Can you work these out from the model? Positions are in its coordinate system, mm. A direction names the side the tool comes from. Coordinates: 2 decimals unless noted, no trailing zeros. Loops run counter-clockwise (first coordinate to the right, second up) from the corner with the lowest first, then second, coordinate; pieces in that order, holes last. Notation, with made-up numbers: M -13.75,-0.5 L 29.25,-0.5 A25 ccw 29.25,25.5 Z; hole C -14,6.25 d6. An arc over 180 degrees is marked long. Answer as a JSON object with one key per item and string values. Group by question number.
Item 1: I'm going to push flat-ended pins straight in: pin 1 Ø5 at (x, y) = (3.5, 69.5) entering from +Z; pin 2 Ø10 at (y, z) = (7, 0) entering from -X; pin 3 Ø5 at (y, z) = (16, 0) entering from +X; pin 4 Ø12 at (x, y) = (-5, 34) entering from -Z. Where does each tip first touch, or does it pass through?
Item 2: Suppose I cut it at C-C (y = 69). Write out the boundary of the cut face in (x, z).
Item 3: Suppose I cut it at B-B (y = 19.5). Write out the boundary of the cut face in (x, z), then the cut area to 3 significant figures.
Item 4: If I drill on line 1 (Y direction, x = 18, z = -5.5); line 2 (Z direction, x = 10, y = 5); line 3 (Y direction, x = -1, z = 9), over which ranges is the centre line in solid material (lowest first)?
Item 5: Which directions (+Z, -Z, +X, -X, +Y, -Y) give clear straight access to the entire face, cutting with the end or side of a thin tool? Please do faces 4 (the cylindrical face through (-0.9, -0.99, -2.86)), 5 (the cylindrical face through (-7.509, 22.717, -23.846)), 6 (the flat face through (15, 45, 0)).
Item 6: We'd pull the mould along X, two halves only. Please class faces 1 (the cylindrical face through (-0.228, 4.93, 11.735)), 2 (the cylindrical face through (12.4, 48.5, -6.5)), 3 (the flat face through (0, -2, 0)): +X half, -X half, draft (parallel to the pull), parting line (faces both ways), or undercut.
Item 7: Suppose I cut it at A-A (x = 0). Write out the boundary of the cut face in (y, z).
```python
from build123d import *

# Parameters (mm, degrees)
SKETCH1_W          = 3
SKETCH1_H          = 2
SKETCH1_W_2        = 4
SKETCH1_H_2        = 7
SKETCH1_W_3        = 10
SKETCH1_H_3        = 28
CHAMFER1_SIZE      = 7
CHAMFER1_SIZE2     = 2.54779164
CHAMFER2_SIZE      = 7
CHAMFER2_SIZE2     = 2.54779164
SKETCH2_R          = 1.75
CUT_EXTRUDE1_DEPTH = 10


with BuildPart() as part:
    # Sketch1 → Revolve1 (revolve)
    with BuildSketch(Plane.XY, mode=Mode.PRIVATE) as revolve1_sk:
        Polygon((0, 45), (0, 0), (3, 0), (25, 0), (25, 45), (14, 45), (4, 45), align=None)
        with Locations((1.5, -1)):
            Rectangle(SKETCH1_W, SKETCH1_H)
        with Locations((2, 48.5)):
            Rectangle(SKETCH1_W_2, SKETCH1_H_2)
        with Locations((9, 48.5)):
            Rectangle(SKETCH1_W_3, SKETCH1_H_2)
        with Locations((2, 66)):
            Rectangle(SKETCH1_W_2, SKETCH1_H_3)
    revolve(revolve1_sk.sketch.rotate(Axis((0, 45, 0), (0, 1, 0)), 90), axis=Axis((0, 45, 0), (0, 1, 0)))

    # Chamfer1
    chamfer1_edges = [part.edges().sort_by_distance(p)[0] for p in [
        (0, 0, 25),
    ]]
    chamfer1_side = [part.faces().sort_by_distance(p)[0] for p in [
        (0, 22.5, 25),
    ]]
    chamfer(chamfer1_edges, length=CHAMFER1_SIZE, length2=CHAMFER1_SIZE2, reference=chamfer1_side[0])

    # Chamfer2
    chamfer2_edges = [part.edges().sort_by_distance(p)[0] for p in [
        (0, 45, 25),
    ]]
    chamfer2_side = [part.faces().sort_by_distance(p)[0] for p in [
        (0, 26, 25),
    ]]
    chamfer(chamfer2_edges, length=CHAMFER2_SIZE, length2=CHAMFER2_SIZE2, reference=chamfer2_side[0])

    # Sketch2 → Cut-Extrude1 (cut)
    with BuildSketch(Plane.XZ):
        with Locations((0, 10)):
            Circle(SKETCH2_R)
        with Locations((10, 0)):
            Circle(SKETCH2_R)
        with Locations((0, -10)):
            Circle(SKETCH2_R)
        with Locations((-10, 0)):
            Circle(SKETCH2_R)
    extrude(amount=-CUT_EXTRUDE1_DEPTH, mode=Mode.SUBTRACT)


solid = part.part
```
From the geometry:
{
 "1": {"pin 1": "z = 3.87", "pin 2": "x = -25", "pin 3": "x = 25", "pin 4": "z = -25"},
 "2": {"outline": "C 0,0 d8"},
 "3": {"outline": "C 0,0 d50", "area": "1,960 mm2"},
 "4": {"line 1": "0 to 45", "line 2": "-22.12 to -1.75, 1.75 to 22.12", "line 3": "10 to 52"},
 "5": {"face 4": "-Y", "face 5": "+Y, -Y", "face 6": "+Y"},
 "6": {"face 1": "undercut", "face 2": "parting line", "face 3": "draft"},
 "7": {"outline": "M -2,-3 L 0,-3 L 0,-8.25 L 10,-8.25 L 10,-11.75 L 0,-11.75 L 0,-22.45 L 7,-25 L 38,-25 L 45,-22.45 L 45,-14 L 52,-14 L 52,-4 L 80,-4 L 80,4 L 52,4 L 52,14 L 45,14 L 45,22.45 L 38,25 L 7,25 L 0,22.45 L 0,11.75 L 10,11.75 L 10,8.25 L 0,8.25 L 0,3 L -2,3 Z"}
}
